from build123d import *

# Parameters (mm, degrees)
SKETCH1_W           = 42
SKETCH1_H           = 42
SKETCH1_R           = 12
SKETCH1_R_2         = 1.6
BOSS_EXTRUDE1_DEPTH = 5
SKETCH3_R           = 3
CUT_EXTRUDE1_DEPTH  = 2


with BuildPart() as part:
    # Sketch1 → Boss-Extrude1 (new body)
    with BuildSketch(Plane(origin=(0, 0, 0), x_dir=(1, 0, 0), z_dir=(0, 1, 0))):
        Rectangle(SKETCH1_W, SKETCH1_H)
        Circle(SKETCH1_R, mode=Mode.SUBTRACT)
        with Locations((15.5, 15.5)):
            Circle(SKETCH1_R_2, mode=Mode.SUBTRACT)
        with Locations((-15.5, 15.5)):
            Circle(SKETCH1_R_2, mode=Mode.SUBTRACT)
        with Locations((-15.5, -15.5)):
            Circle(SKETCH1_R_2, mode=Mode.SUBTRACT)
        with Locations((15.5, -15.5)):
            Circle(SKETCH1_R_2, mode=Mode.SUBTRACT)
        Polygon((-31, -21), (-21, -21), (-21, -7), (-27, -7), (-31, -11), align=None)
        with Locations((-26, -14)):
            Circle(SKETCH1_R_2, mode=Mode.SUBTRACT)
        Polygon((21, -7), (21, -21), (31, -21), (31, -11), (27, -7), align=None)
        with Locations((26, -14)):
            Circle(SKETCH1_R_2, mode=Mode.SUBTRACT)
        Polygon((-7, 29), (-11, 21), (7, 21), (3, 29), align=None)
        with Locations((-2, 25)):
            Circle(SKETCH1_R_2, mode=Mode.SUBTRACT)
        Polygon((21, 21), (21, -7), (27, -7), (31, -11), align=None)
        Polygon((-7, 29), (-21, 21), (-11, 21), align=None)
        Polygon((7, 21), (21, 21), (3, 29), align=None)
    extrude(amount=BOSS_EXTRUDE1_DEPTH)

    # Sketch3 → Cut-Extrude1 (cut)
    with BuildSketch(Plane(origin=(0, 5, 0), x_dir=(1, 0, 0), z_dir=(0, 1, 0))):
        with Locations((-15.5, 15.5)):
            Circle(SKETCH3_R)
        with Locations((15.5, 15.5)):
            Circle(SKETCH3_R)
        with Locations((15.5, -15.5)):
            Circle(SKETCH3_R)
        with Locations((-15.5, -15.5)):
            Circle(SKETCH3_R)
    extrude(amount=-CUT_EXTRUDE1_DEPTH, mode=Mode.SUBTRACT)


solid = part.part
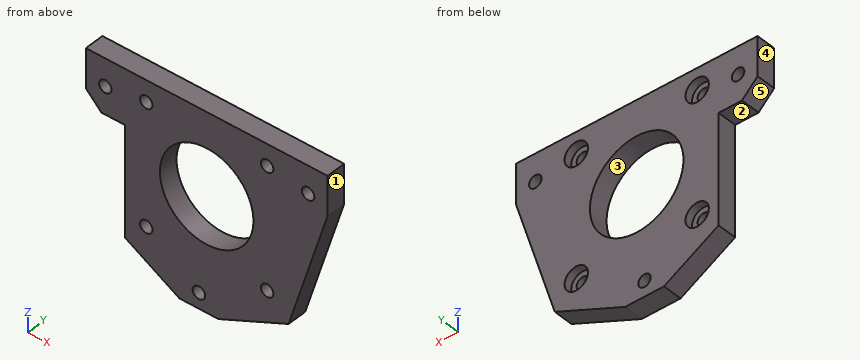
Verification items for the finished model (mm, model axes). Face numbers are marked on the shaded views. A direction names the side the tool comes from. Coordinates: 2 decimals unless noted, no trailing zeros. Order: outer loops, then holes, each group sorted by start corner. A loop starts at its lowest first (then second) coordinate and runs counter-clockwise, first axis right, second up. Notation, with made-up numbers: M 17.5,-33 L 45.5,-33 A20 ccw 45.5,-19 Z; hole C -23,-8.5 d2. An arc over 180 degrees is marked long. One line per item, written item: value. Start each with the question number.
Item 1: Mould release check, pull along Z, two halves, no side actions. Record for the marked faces 3, 4 and 5: pulls with the +Z half, pulls with the -Z half, needs draft (parallel to the pull), parting line crosses it, or undercut.
Item 2: Sectioned sample at B-B on x = 26. Record the cut outline in (y, z), then the cut area to 3 significant figures.
Item 3: Sectioned sample at A-A on z = -25. Record the cut outline in (x, y), then the cut area to 3 significant figures.
Item 4: Depth check by flat-ended pin: P1, Ø2.5, axis at x = -25, y = 2, coming from the -Z side; P2, Ø1.5, axis at y = 1.5, z = -18, coming from the -X side; P3, Ø4, axis at x = 15.5, z = -15.5, coming from the +Y side. Enter the tip coordinate at first touch or a pass-through.
Item 5: Sectioned sample at D-D on x = -15.5. Record the cut outline in (y, z).
Item 6: Thickness scan on probe 1 along X at (y, z) = (3.55, -15.5); probe 2 along Z at (x, y) = (-15.5, 4.45); probe 3 along Z at (x, y) = (-2, 3.9). Record the ranges inside material, lowest first.
Item 7: Access from +Z, -Z, +X, -X, +Y, -Y to the whole of each face (thin tool, end or side, straight path). Record for the marked faces 1 and 2.
Item 8: Sectioned sample at C-C on y = 4. Give the number of separate pieces and of enclosed holes in the cut face, then the cut area to 3 significant figures.
Calculated:
1. face 3: undercut
1. face 4: needs draft
1. face 5: pulls with the -Z half
2. outline: M 0,-5 L 5,-5 L 5,12.4 L 0,12.4 Z; M 0,15.6 L 5,15.6 L 5,21 L 0,21 Z
2. area: 114 mm^2
3. outline: M -14,0 L -3.6,0 L -3.6,5 L -14,5 Z; M -0.4,0 L 12,0 L 12,5 L -0.4,5 Z
3. area: 114 mm^2
4. P1: z = 7
4. P2: x = -21
4. P3: y = 3
5. outline: M 0,-24.14 L 5,-24.14 L 5,-18.5 L 3,-18.5 L 3,-17.1 L 0,-17.1 Z; M 0,-13.9 L 3,-13.9 L 3,-12.5 L 5,-12.5 L 5,12.5 L 3,12.5 L 3,13.9 L 0,13.9 Z; M 0,17.1 L 3,17.1 L 3,18.5 L 5,18.5 L 5,21 L 0,21 Z
6. probe 1: -21 to -18.5, -12.5 to 12.5, 18.5 to 22.72
6. probe 2: -24.14 to -18.5, -12.5 to 12.5, 18.5 to 21
6. probe 3: -29 to -26.6, -23.4 to -11.83, 11.83 to 21
7. face 1: +Z, -Z, +X, +Y, -Y
7. face 2: -Z, -X, +Y, -Y
8. separate pieces: 1
8. enclosed holes: 8
8. area: 1,770 mm^2
